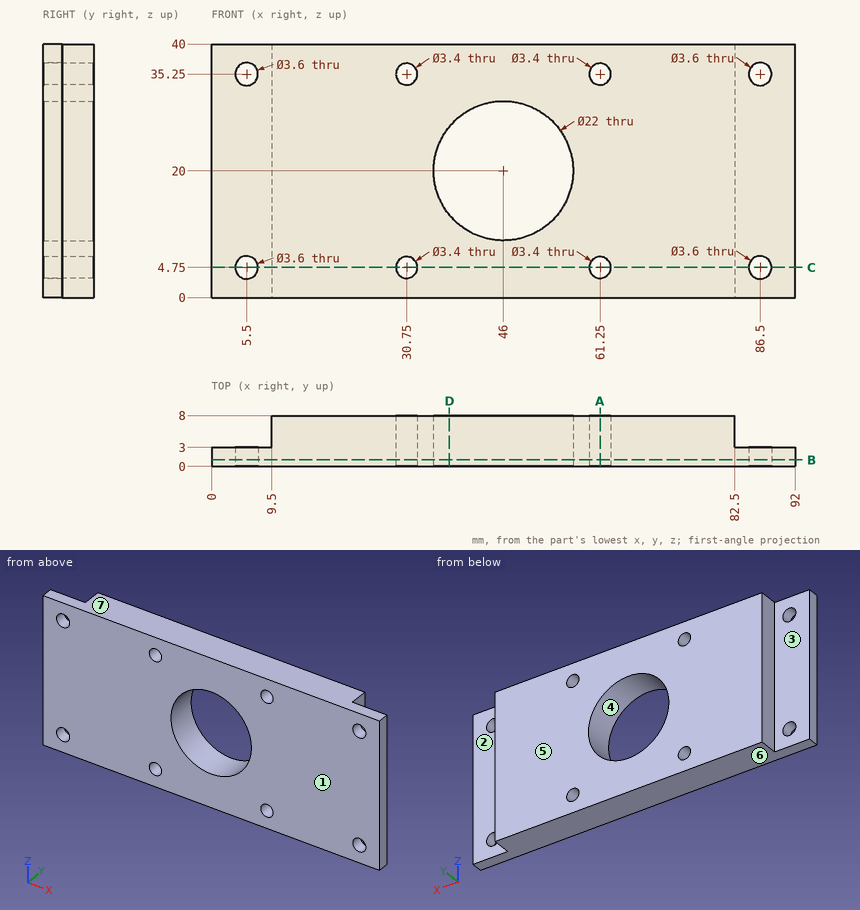
Design review of the part shown in the three views and the two pictorial views. Dimensions are in mm from the part's minimum x, y and z. A direction names the side the tool comes from. Round coordinates to 2 decimals unless told otherwise and drop trailing zeros. Write each loop counter-clockwise with the first axis right and the second up, starting at its lowest first coordinate (ties: lowest second). Pieces come first, ordered by that corner, then holes. Notation, with made-up numbers: (83.5, 18.5) - (101.5, 18.5) arc R22 cw to (101.5, 54.5) - close; hole circle Ø8 at (84.25, 65.25). An arc over 180 degrees is marked (long way). Write item = value, one per line. Start each with the question number.
1. Consider section A-A on x = 61.25. State the section outline as (y, z) points, plus the area to 3 significant figures.
2. For pin 1 Ø3 at (x, z) = (15.5, 13) entering from -Y; pin 2 Ø3 at (x, z) = (86.5, 35.25) entering from +Y; pin 3 Ø1 at (y, z) = (5.5, 8.5) entering from -X; pin 4 Ø1 at (y, z) = (5.5, 11.5) entering from +X, all flat-tipped, find the tip position at first contact; note any pin that passes through.
3. Consider section B-B on y = 1. Give the number of separate pieces and of enclosed holes in the cut face, plus the area to 3 significant figures.
4. Consider section C-C on z = 4.75. State the section outline as (x, y) points.
5. For the marked faces 1, 2 and 3, list the 3-axis set-ups (+Z, -Z, +X, -X, +Y, -Y) from which the entire face can be reached by the end or side of a thin tool; tool diameter is ignored.
6. Draft analysis for pull direction Z (two halves, no side actions). For the marked faces 4, 5, 6 and 7, state which applies: released by +Z, released by -Z, zero draft, split by the parting line, or undercut.
7. Consider section D-D on x = 37.5. State the section outline as (y, z) points.
8. Wall thickness on L1, parallel to X at y = 1.95, z = 4.75; L2, parallel to Z at x = 61.25, y = 2.5; L3, parallel to X at y = 5.5, z = 35.5: over which ranges is each line inside the solid? List them lowest first.
Evaluation:
q1.outline = (0, 0) - (8, 0) - (8, 3.05) - (0, 3.05) - close; (0, 6.45) - (8, 6.45) - (8, 33.55) - (0, 33.55) - close; (0, 36.95) - (8, 36.95) - (8, 40) - (0, 40) - close
q1.area = 266 mm2
q2.pin_1 = 0
q2.pin_2 = through
q2.pin_3 = 9.5
q2.pin_4 = 82.5
q3.separate_pieces = 1
q3.enclosed_holes = 9
q3.area = 3,220 mm2
q4.outline = (0, 0) - (3.7, 0) - (3.7, 3) - (0, 3) - close; (7.3, 0) - (29.05, 0) - (29.05, 8) - (9.5, 8) - (9.5, 3) - (7.3, 3) - close; (32.45, 0) - (59.55, 0) - (59.55, 8) - (32.45, 8) - close; (62.95, 0) - (84.7, 0) - (84.7, 3) - (82.5, 3) - (82.5, 8) - (62.95, 8) - close; (88.3, 0) - (92, 0) - (92, 3) - (88.3, 3) - close
q5.face_1 = +Z, -Z, +X, -X, -Y
q5.face_2 = +Z, -Z, +X, +Y
q5.face_3 = +Z, -Z, -X, +Y
q6.face_4 = undercut
q6.face_5 = zero draft
q6.face_6 = released by -Z
q6.face_7 = released by +Z
q7.outline = (0, 0) - (8, 0) - (8, 13.02) - (0, 13.02) - close; (0, 26.98) - (8, 26.98) - (8, 40) - (0, 40) - close
q8.L1 = 0 to 3.7, 7.3 to 29.05, 32.45 to 59.55, 62.95 to 84.7, 88.3 to 92
q8.L2 = 0 to 3.05, 6.45 to 33.55, 36.95 to 40
q8.L3 = 9.5 to 29.07, 32.43 to 59.57, 62.93 to 82.5
